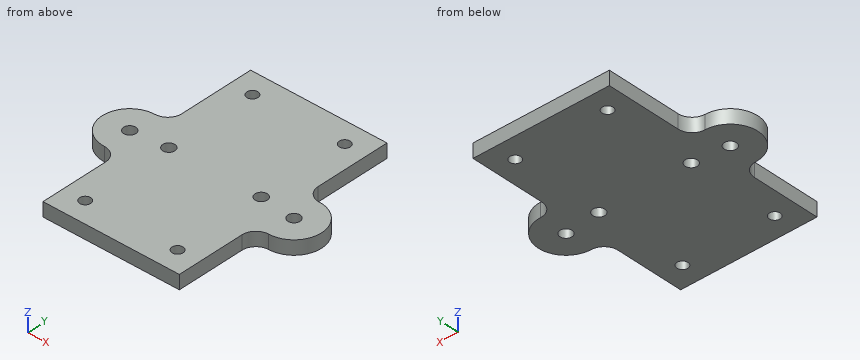
Autodesk Inventor part; units mm, degrees
ref_plane "YZ Plane" through (0, 0, 0) normal (1, 0, 0) x (0, 1, 0)
ref_plane "XZ Plane" through (0, 0, 0) normal (0, 1, 0) x (-1, 0, 0)
ref_plane "XY Plane" through (0, 0, 0) normal (0, 0, 1) x (1, 0, 0)
sketch "Sketch1" plane through (0, 0, 0) normal (0, 0, 1) x (1, 0, 0)
  circle A0 centre (-610.4613, 17.8) radius 2.5
  circle A1 centre (-610.4613, 17.8) radius 9.9 construction
  circle A2 centre (-652.4613, 17.8) radius 2.5
  circle A3 centre (-652.4613, 17.8) radius 9.9 construction
  circle A4 centre (-610.4613, -65) radius 2.5
  circle A5 centre (-610.4613, -65) radius 9.9 construction
  circle A6 centre (-652.4613, -65) radius 2.5
  circle A7 centre (-652.4613, -65) radius 9.9 construction
  line L0 (-610.4613, -65) -> (-652.4613, -65) construction
  line L1 (-652.4613, -65) -> (-652.4613, 17.8) construction
  line L2 (-652.4613, 17.8) -> (-610.4613, 17.8) construction
  line L3 (-610.4613, 17.8) -> (-610.4613, -65) construction
  line L4 (-662.4613, -75) -> (-600.4613, -75)
  line L5 (-600.4613, -75) -> (-600.4613, 27.8)
  line L6 (-600.4613, 27.8) -> (-662.4613, 27.8)
  line L7 (-662.4613, 27.8) -> (-662.4613, -75)
  point P0 (0, 0)
  dimension "d0" = 10
extrude "Extrusion1" add sketch "Sketch1" along normal blind 6.35
sketch "Sketch2" plane through (0, 0, 6.35) normal (0, 0, 1) x (1, 0, 0)
  circle A0 centre (-610.4613, 17.8) radius 2.5
  circle A1 centre (-610.4613, -65) radius 2.5
  circle A2 centre (-652.4613, -65) radius 2.5
  circle A3 centre (-652.4613, 17.8) radius 2.5
  circle A4 centre (-652.4613, 17.8) radius 2.5
  line L0 (-652.4613, 17.8) -> (-652.4613, -65) construction
  circle A5 centre (-610.4613, 17.8) radius 2.5
  circle A6 centre (-610.4613, -65) radius 2.5
  line L1 (-610.4613, 17.8) -> (-610.4613, -65) construction
  circle A7 centre (-610.4613, -23.6) radius 2.75
  circle A8 centre (-652.4613, -23.6) radius 2.75
  point P0 (0, 0)
  dimension "d3" = 5.5
extrude "Extrusion2" cut sketch "Sketch2" against normal blind 25.4 contours A7 | A8
sketch "Sketch3" plane through (0, 0, 6.35) normal (0, 0, 1) x (1, 0, 0)
  line L0 (-688.334, -23.6) -> (-567.3626, -23.6) construction
  line L1 (-600.4613, -75) -> (-600.4613, 27.8) construction
  line L2 (-662.4613, 27.8) -> (-662.4613, -75) construction
  line L3 (-594.1113, -75) -> (-594.1113, 27.8) construction
  line L4 (-668.8113, 24.7) -> (-668.8113, -75) construction
  circle A0 centre (-668.8113, -25.15) radius 2.75
  arc A1 (-668.8113, -12.6221) -> (-668.8113, -37.6779) centre (-668.8113, -25.15) ccw
  line L5 (-600.4613, -75) -> (-600.4613, 27.8)
  arc A2 (-662.4613, -44.0279) -> (-668.8113, -37.6779) centre (-668.8113, -44.0279) ccw
  arc A3 (-668.8113, -12.6221) -> (-662.4613, -6.2721) centre (-668.8113, -6.2721) ccw
  line L6 (-668.8113, -6.2721) -> (-662.4613, -6.2721) construction
  line L7 (-668.8113, -6.2721) -> (-668.8113, -12.6221) construction
  line L8 (-600.4613, 27.8) -> (-662.4613, 27.8) construction
  line L9 (-631.4613, 27.8) -> (-631.4613, -75) construction
  line L10 (-662.4613, -75) -> (-600.4613, -75) construction
  circle A4 centre (-594.1113, -25.15) radius 2.75
  arc A5 (-594.1113, -37.6779) -> (-594.1113, -12.6221) centre (-594.1113, -25.15) ccw
  arc A6 (-594.1113, -37.6779) -> (-600.4613, -44.0279) centre (-594.1113, -44.0279) ccw
  arc A7 (-600.4613, -6.2721) -> (-594.1113, -12.6221) centre (-594.1113, -6.2721) ccw
  line L11 (-594.1113, -6.2721) -> (-600.4613, -6.2721) construction
  line L12 (-594.1113, -6.2721) -> (-594.1113, -12.6221) construction
  line L13 (-662.4613, -6.2721) -> (-662.4613, -44.0279) construction
  line L14 (-662.4613, -6.2721) -> (-662.4613, -44.0279)
  line L15 (-600.4613, -44.0279) -> (-600.4613, -6.2721)
  point P0 (0, 0)
  point P1 (-574.5885, -23.6)
  dimension "d6" = 6.35
  dimension "d7" = 6.35
  dimension "d9" = 6.35
  dimension "d10" = 90
  dimension "d11" = 6.35
  dimension "d14" = 1.55
  dimension "d15" = 51.4
extrude "Extrusion3" add sketch "Sketch3" against normal up to surface (6.35 mm away)
properties part number "yCarraige"
The listing builds one solid part. Answer for the finished solid, in the listing's coordinates (mm). Give positions to 0.01 mm unless a question says otherwise; leave off trailing zeros. Order: outer loops, then holes, each group sorted by start corner. A loop starts at its lowest first (then second) coordinate and runs counter-clockwise, first axis right, second up. Notation, with made-up numbers: (1, -38) - (22, -38) arc R30 ccw to (22, -3) - close; hole circle Ø3 at (52, 1). An arc over 180 degrees is marked (long way). Answer in a Markdown table with one row per item. Add a question column.
Q1. The part is cut by section C-C (y = -25.15). Determine the outline of the cut face in (x, z), then the cut area to 3 significant figures.
Q2. Find the intervals of material crossed by line 1 along X through (y, z) = (18, 1); line 2 along Y through (x, z) = (-653, 5); line 3 along Y through (x, z) = (-651, 6), in increasing order. Write a range as [from, to].
Q3. The part is cut by section B-B (z = 2). Give the number of separate pieces and of enclosed holes in the cut face, then the cut area to 3 significant figures.
Q4. The part is cut by section A-A (y = 17.8). Determine the outline of the cut face in (x, z), then the cut area to 3 significant figures.
Q5. Given P1, Ø1, axis at x = -599, z = 1, coming from the -Y side; P2, Ø2, axis at y = 12, z = 2, coming from the -X side, each flat-ended and moving along its own axis, determine where each tip first touches the part or whether it passes through.
Q6. The part is cut by section D-D (y = -49). Determine the outline of the cut face in (x, z), then the cut area to 3 significant figures.
Determined:
| question | item | result |
|---|---|---|
| 1 | outline | (-681.34, 0) - (-671.56, 0) - (-671.56, 6.35) - (-681.34, 6.35) - close; (-666.06, 0) - (-654.73, 0) - (-654.73, 6.35) - (-666.06, 6.35) - close; (-650.19, 0) - (-612.73, 0) - (-612.73, 6.35) - (-650.19, 6.35) - close; (-608.19, 0) - (-596.86, 0) - (-596.86, 6.35) - (-608.19, 6.35) - close; (-591.36, 0) - (-581.58, 0) - (-581.58, 6.35) - (-591.36, 6.35) - close |
| 1 | area | 506 mm² |
| 2 | line 1 | x = [-662.46, -654.95], [-649.97, -612.95], [-607.97, -600.46] |
| 2 | line 2 | y = [-75, -67.44], [-62.56, -26.3], [-20.9, 15.36], [20.24, 27.8] |
| 2 | line 3 | y = [-75, -67.03], [-62.97, -25.93], [-21.27, 15.77], [19.83, 27.8] |
| 3 | separate pieces | 1 |
| 3 | enclosed holes | 8 |
| 3 | area | 7,050 mm² |
| 4 | outline | (-662.46, 0) - (-654.96, 0) - (-654.96, 6.35) - (-662.46, 6.35) - close; (-649.96, 0) - (-612.96, 0) - (-612.96, 6.35) - (-649.96, 6.35) - close; (-607.96, 0) - (-600.46, 0) - (-600.46, 6.35) - (-607.96, 6.35) - close |
| 4 | area | 330 mm² |
| 5 | P1 | stops at y = -40.67 |
| 5 | P2 | stops at x = -662.46 |
| 6 | outline | (-662.46, 0) - (-600.46, 0) - (-600.46, 6.35) - (-662.46, 6.35) - close |
| 6 | area | 394 mm² |
